Could you check a few things on this model? Use its own coordinates, in mm. Face numbers are marked on the shaded views. A direction names the side the tool comes from. Coordinates: 2 decimals unless noted, no trailing zeros. Write each loop counter-clockwise with the first axis right and the second up, starting at its lowest first coordinate (ties: lowest second). Pieces come first, ordered by that corner, then holes.
```python
from build123d import *

# Parameters (mm, degrees)
SKETCH_8_W                = 70
SKETCH_8_H                = 30
EXTRUDE_3_DEPTH           = 34.57
SKETCH_9_W                = 30
SKETCH_9_H                = 14.57
SKETCH_9_W_2              = 20
CUT_EXTRUDE_3_DEPTH       = 67.664217758
OTHER_1_OUTLINE_R         = 5.5
OTHER_1_DEPTH             = 5
HOLE_WIZARD_2_D           = 4.5
HOLE_WIZARD_2_DEPTH       = 10
HOLE_WIZARD_2_CBORE_D     = 8
HOLE_WIZARD_2_CBORE_DEPTH = 4.6
BACK_REACH                = 69.458
SKETCH_16_W               = 70
SKETCH_16_H               = 8.975361008
MM_1_D                    = 4
MM_1_DEPTH                = 5
MM_1_TIP                  = 1.201721238
CUT_EXTRUDE_5_DEPTH       = 5
SKETCH_24_W               = 5
SKETCH_24_H               = 21.024638992
SKETCH_24_W_2             = 20
CUT_EXTRUDE_6_DEPTH       = 10
HOLE_WIZARD_3_D           = 6.6
HOLE_WIZARD_3_DEPTH       = 10
HOLE_WIZARD_3_CBORE_D     = 11
HOLE_WIZARD_3_CBORE_DEPTH = 6.8
FILLET_1_R                = 2
SKETCH_29_W               = 10
SKETCH_29_H               = 2
EXTRUDE_5_DEPTH           = 2.329281552
FILLET_3_R                = 2
CUT_EXTRUDE_7_DEPTH       = 0.5
EXTRUDE_START             = 5.016506594
EXTRUDE_6_DEPTH           = 5.016506594


# Read off the part's stored shape, not the designer's step: 孔1
with BuildPart() as part:
    # 草图8 → 凸台-拉伸3 (new body)
    with BuildSketch(Plane(origin=(0, 0, 0), x_dir=(1, 0, 0), z_dir=(0, 1, 0))):
        with Locations((13.466824006, -16.724598186)):
            Rectangle(SKETCH_8_W, SKETCH_8_H)
    extrude(amount=EXTRUDE_3_DEPTH)

    # 草图9 → 切除-拉伸3 (cut, through all)
    with BuildSketch(Plane.XY.offset(31.724598186)):
        with Locations((-6.533175994, 17.285)):
            Rectangle(SKETCH_9_W, SKETCH_9_H)
        with Locations((38.466824006, 17.285)):
            Rectangle(SKETCH_9_W_2, SKETCH_9_H)
    extrude(amount=-CUT_EXTRUDE_3_DEPTH, mode=Mode.SUBTRACT)

    # 孔1 outline → 孔1 (cut)
    with BuildSketch(Plane(origin=(0, 0, 0), x_dir=(1, 0, 0), z_dir=(0, 1, 0))):
        with Locations((-1.533175994, -21.724598186)):
            Circle(OTHER_1_OUTLINE_R)
    extrude(amount=OTHER_1_DEPTH, mode=Mode.SUBTRACT)

    # 打孔尺寸(%根据)内六角圆柱头螺钉的类型2
    with Locations(Plane(origin=(-1.533175994, 10, 21.724598186), x_dir=(1, 0, 0), z_dir=(0, 1, 0))):
        with Locations((0, 0)):
            CounterBoreHole(HOLE_WIZARD_2_D / 2, HOLE_WIZARD_2_CBORE_D / 2, HOLE_WIZARD_2_CBORE_DEPTH, depth=HOLE_WIZARD_2_DEPTH)

    # back: up to this face of the body (flat: up to its plane)
    back_end = Plane(part.part.faces().sort_by_distance((-6.533175994, 24.57, 16.724598186))[0])
    # 草图16 → back (cut, up to the picked face)
    with BuildSketch(Plane(origin=(0, 0, 0), x_dir=(1, 0, 0), z_dir=(0, 1, 0)), mode=Mode.PRIVATE) as back_sk1:
        with Locations((13.466824006, -6.21227869)):
            Rectangle(SKETCH_16_W, SKETCH_16_H)
    back_tool1 = split(extrude(back_sk1.sketch, amount=BACK_REACH, mode=Mode.PRIVATE), bisect_by=back_end, keep=Keep.BOTH, mode=Mode.PRIVATE)
    add(back_tool1.solids().sort_by(Axis((13.466824, 0, 6.212279), (0, 1, 0)))[0], mode=Mode.SUBTRACT)

    # 大小mm 暗销孔1
    with Locations(Plane(origin=(-1.533175994, 34.57, 11.724598186), x_dir=(0, 0, 1), z_dir=(0, 1, 0))):
        with Locations((0, 0)):
            Hole(MM_1_D / 2, depth=MM_1_DEPTH)
            with Locations((0, 0, -(MM_1_DEPTH + MM_1_TIP / 2))):  # 118° drill point
                Cone(0, MM_1_D / 2, MM_1_TIP, mode=Mode.SUBTRACT)

    # 草图23 → 切除-拉伸5 (cut)
    with BuildSketch(Plane.XZ.offset(-34.57)):
        with BuildLine():
            Line((28.966824006, 9.724598186), (27.966824006, 9.724598186))
            ThreePointArc((27.966824006, 9.724598186), (25.966824006, 11.724598186), (27.966824006, 13.724598186))
            Line((27.966824006, 13.724598186), (28.966824006, 13.724598186))
            ThreePointArc((28.966824006, 13.724598186), (30.966824006, 11.724598186), (28.966824006, 9.724598186))
        make_face()
    extrude(amount=CUT_EXTRUDE_5_DEPTH, mode=Mode.SUBTRACT)

    # 草图24 → 切除-拉伸6 (cut)
    with BuildSketch(Plane(origin=(0, 0, 0), x_dir=(1, 0, 0), z_dir=(0, 1, 0))):
        with Locations((-19.033175994, -21.21227869)):
            Rectangle(SKETCH_24_W, SKETCH_24_H)
        with Locations((38.466824006, -21.21227869)):
            Rectangle(SKETCH_24_W_2, SKETCH_24_H)
    extrude(amount=CUT_EXTRUDE_6_DEPTH, mode=Mode.SUBTRACT)

    # 打孔尺寸(%根据)内六角圆柱头螺钉的类型3
    with Locations(Plane(origin=(-11.533175994, 24.57, 11.724598186), x_dir=(0, 0, -1), z_dir=(0, -1, 0))):
        with Locations((0, 0), (0, 50)):
            CounterBoreHole(HOLE_WIZARD_3_D / 2, HOLE_WIZARD_3_CBORE_D / 2, HOLE_WIZARD_3_CBORE_DEPTH, depth=HOLE_WIZARD_3_DEPTH)

    # 圆角1
    fillet_1_edges = [part.edges().sort_by_distance(p)[0] for p in [
        (-16.533175994, 0, 21.21227869),
        (-16.533175994, 10, 21.21227869),
        (28.466824006, 0, 21.21227869),
        (-21.533175994, 24.57, 16.724598186),
        (48.466824006, 24.57, 16.724598186),
        (8.466824006, 24.57, 21.21227869),
        (28.466824006, 24.57, 21.21227869),
    ]]
    fillet(fillet_1_edges, radius=FILLET_1_R)

    # 草图29 → 凸台-拉伸5 (add)
    with BuildSketch(Plane(origin=(0, 0, 10.699959194), x_dir=(-1, 0, 0), z_dir=(0, 0, -1))):
        with Locations((0, -1)):
            Rectangle(SKETCH_29_W, SKETCH_29_H)
    extrude(amount=-EXTRUDE_5_DEPTH)

    # 圆角3
    fillet_3_edges = [part.edges().sort_by_distance(p)[0] for p in [
        (-5, -2, 11.86459997),
        (5, -2, 11.86459997),
    ]]
    fillet(fillet_3_edges, radius=FILLET_3_R - 0.0001)  # a hair under: the kernel refuses the full size

    # 草图30 → 切除-拉伸7 (cut)
    with BuildSketch(Plane.XY.offset(31.724598186)):
        with BuildLine():
            Line((-14.533175994, 0), (26.466824006, 0))
            ThreePointArc((26.466824006, 0), (27.881037569, 0.585786438), (28.466824006, 2))
            Line((28.466824006, 2), (28.466824006, 22.57))
            ThreePointArc((28.466824006, 22.57), (29.052610444, 23.984213562), (30.466824006, 24.57))
            Line((30.466824006, 24.57), (46.466824006, 24.57))
            ThreePointArc((46.466824006, 24.57), (47.881037569, 25.155786438), (48.466824006, 26.57))
            Line((48.466824006, 26.57), (48.466824006, 34.57))
            Line((48.466824006, 34.57), (-21.533175994, 34.57))
            Line((-21.533175994, 34.57), (-21.533175994, 26.57))
            ThreePointArc((-21.533175994, 26.57), (-20.947389556, 25.155786438), (-19.533175994, 24.57))
            Line((-19.533175994, 24.57), (6.466824006, 24.57))
            ThreePointArc((6.466824006, 24.57), (7.881037569, 23.984213562), (8.466824006, 22.57))
            Line((8.466824006, 22.57), (8.466824006, 10))
            Line((8.466824006, 10), (-14.533175994, 10))
            ThreePointArc((-14.533175994, 10), (-15.947389556, 9.414213562), (-16.533175994, 8))
            Line((-16.533175994, 8), (-16.533175994, 2))
            ThreePointArc((-16.533175994, 2), (-15.947389556, 0.585786438), (-14.533175994, 0))
        make_face()
    extrude(amount=-CUT_EXTRUDE_7_DEPTH, mode=Mode.SUBTRACT)

    # 草图31 → 凸台-拉伸6 (add)
    with BuildSketch(Plane.XY.offset(31.224598186).offset(EXTRUDE_START)):
        with BuildLine():
            Line((-14.533175994, 0), (26.466824006, 0))
            ThreePointArc((26.466824006, 0), (27.881037569, 0.585786438), (28.466824006, 2))
            Line((28.466824006, 2), (28.466824006, 22.57))
            ThreePointArc((28.466824006, 22.57), (29.052610444, 23.984213562), (30.466824006, 24.57))
            Line((30.466824006, 24.57), (46.466824006, 24.57))
            ThreePointArc((46.466824006, 24.57), (47.881037569, 25.155786438), (48.466824006, 26.57))
            Line((48.466824006, 26.57), (48.466824006, 34.57))
            Line((48.466824006, 34.57), (-21.533175994, 34.57))
            Line((-21.533175994, 34.57), (-21.533175994, 26.57))
            ThreePointArc((-21.533175994, 26.57), (-20.947389556, 25.155786438), (-19.533175994, 24.57))
            Line((-19.533175994, 24.57), (6.466824006, 24.57))
            ThreePointArc((6.466824006, 24.57), (7.881037569, 23.984213562), (8.466824006, 22.57))
            Line((8.466824006, 22.57), (8.466824006, 10))
            Line((8.466824006, 10), (-14.533175994, 10))
            ThreePointArc((-14.533175994, 10), (-15.947389556, 9.414213562), (-16.533175994, 8))
            Line((-16.533175994, 8), (-16.533175994, 2))
            ThreePointArc((-16.533175994, 2), (-15.947389556, 0.585786438), (-14.533175994, 0))
        make_face()
    extrude(amount=-EXTRUDE_6_DEPTH)


solid = part.part
```
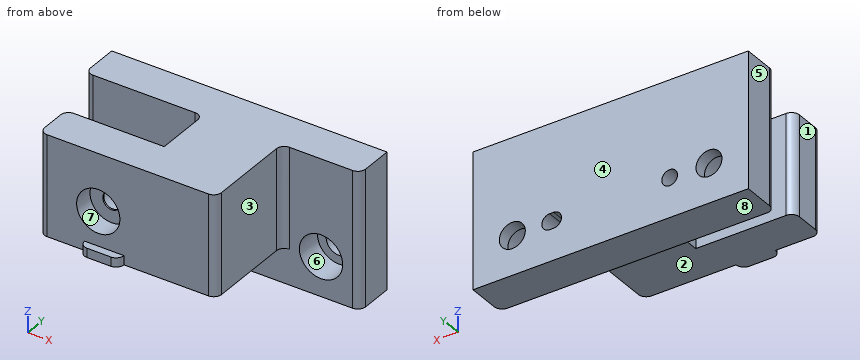
1. For pin 1 (9 mm diameter, centred on x = -1.53, z = 21.72, fed in from -Y); pin 2 (9 mm diameter, centred on x = 38.47, z = 11.72, fed in from +Y); pin 3 (8 mm diameter, centred on x = 11, y = 5, fed in from -Z); pin 4 (2 mm diameter, centred on x = 27.5, z = 11, fed in from +Y), each with a flat end and sliding along its axis, tell me the tip position at first contact or that it passes through.
Verdict:
pin 1: stops at y = 5
pin 2: stops at y = 34.57
pin 3: stops at z = 10.7
pin 4: stops at y = 29.57
2. I want a section at B-B on z = 34. Please give me the cut outline in (x, y).
Verdict:
outline: (-21.53, 26.57) arc R2 ccw to (-19.53, 24.57) - (6.47, 24.57) arc R2 cw to (8.47, 22.57) - (8.47, 10) - (-14.53, 10) arc R2 ccw to (-16.53, 8) - (-16.53, 2) arc R2 ccw to (-14.53, 0) - (26.47, 0) arc R2 ccw to (28.47, 2) - (28.47, 22.57) arc R2 cw to (30.47, 24.57) - (46.47, 24.57) arc R2 ccw to (48.47, 26.57) - (48.47, 34.57) - (-21.53, 34.57) - close
3. If we mould it in two halves opening along X, with no side actions, what happens to the marked faces 5, 6, 7 and 8? For each: pulls with the +X half, pulls with the -X half, needs draft (parallel to the pull), parting line crosses it, or undercut.
Verdict:
face 5: pulls with the -X half
face 6: undercut
face 7: undercut
face 8: needs draft
4. I want a section at A-A on x = 19. Please give me the cut outline in (y, z), plus the area to 3 significant figures.
Verdict:
outline: (0, 10.7) - (24.57, 10.7) - (24.57, 1.72) - (34.57, 1.72) - (34.57, 36.24) - (0, 36.24) - close
area: 973 mm2
5. On a 3-axis mill with a long thin cutter (end or side, diameter ignored), from which of +Z, -Z, +X, -X, +Y, -Y can I reach the whole of each face in a straight line? I mean the marked faces 1, 2, 3 and 4. Say none if no direction works.
Verdict:
face 1: +Z, -Z, -X, -Y
face 2: -Z, +X, -X, -Y
face 3: +Z, -Z, +X, -Y
face 4: +Z, -Z, +X, -X, +Y
6. I want a section at C-C on y = 4. Please give me the cut outline in (x, z).
Verdict:
outline: (-16.53, 10.7) - (28.47, 10.7) - (28.47, 36.24) - (-16.53, 36.24) - close; hole circle Ø11 at (-1.53, 21.72)
7. I want a section at D-D on x = 41. Please give me the cut outline in (y, z), plus the area to 3 significant figures.
Verdict:
outline: (24.57, 1.72) - (34.57, 1.72) - (34.57, 9.61) - (31.37, 9.61) - (31.37, 6.84) - (24.57, 6.84) - close; (24.57, 16.61) - (31.37, 16.61) - (31.37, 13.84) - (34.57, 13.84) - (34.57, 36.24) - (24.57, 36.24) - close
area: 265 mm2
8. Please list where these lines run through material, in increasing order: line 1 along X through (y, z) = (28.5, 8); line 2 along X through (y, z) = (30, 9.5); line 3 along Y through (x, z) = (4.5, 34).
Verdict:
line 1: x = -21.53 to -15.58, -7.49 to 34.42, 42.51 to 48.47
line 2: x = -21.53 to -16.56, -6.5 to 33.44, 43.5 to 48.47
line 3: y = 0 to 10, 24.57 to 34.57
